Geometry: final body of the model. Coordinates: model frame, mm. Give positions to 0.01 mm unless a question says otherwise; leave off trailing zeros. Write each loop counter-clockwise with the first axis right and the second up, starting at its lowest first coordinate (ties: lowest second). Pieces come first, ordered by that corner, then holes.
from build123d import *

# Parameters (mm, degrees)
SKETCH_1_W      = 228
SKETCH_1_H      = 84
SKETCH_1_R      = 5
SKETCH_1_R_2    = 1.65
SKETCH_1_R_3    = 2.15
EXTRUDE_1_DEPTH = 1


with BuildPart() as part:
    # Эскиз1 → Вытянуть1 (new body)
    with BuildSketch(Plane.XY):
        Rectangle(SKETCH_1_W, SKETCH_1_H)
        with Locations((74, -2)):
            Circle(SKETCH_1_R, mode=Mode.SUBTRACT)
        with Locations((74, -12)):
            Circle(SKETCH_1_R_2, mode=Mode.SUBTRACT)
        with Locations((62, -2)):
            Circle(SKETCH_1_R, mode=Mode.SUBTRACT)
        with Locations((62, -12)):
            Circle(SKETCH_1_R_2, mode=Mode.SUBTRACT)
        with Locations((50, -2)):
            Circle(SKETCH_1_R, mode=Mode.SUBTRACT)
        with Locations((50, -12)):
            Circle(SKETCH_1_R_2, mode=Mode.SUBTRACT)
        with Locations((38, -2)):
            Circle(SKETCH_1_R, mode=Mode.SUBTRACT)
        with Locations((38, -12)):
            Circle(SKETCH_1_R_2, mode=Mode.SUBTRACT)
        with Locations((107, 32)):
            Circle(SKETCH_1_R_3, mode=Mode.SUBTRACT)
        with Locations(Location((-107, 32, 0), (0, 0, 180))):
            Circle(SKETCH_1_R_3, mode=Mode.SUBTRACT)
        with Locations((-107, -32)):
            Circle(SKETCH_1_R_3, mode=Mode.SUBTRACT)
        with Locations(Location((107, -32, 0), (0, 0, 180))):
            Circle(SKETCH_1_R_3, mode=Mode.SUBTRACT)
    extrude(amount=EXTRUDE_1_DEPTH)


solid = part.part
Q1. Pull-direction query (Y, two-part tool) for faces 1 (the cylindrical face through (108.585, -33.453, 0.493)), 2 (the flat face through (-2, 1, 0)); classes: released by +Y, released by -Y, zero draft, split by the parting line, or undercut.
Filled sheet:
face 1: undercut
face 2: zero draft
Q2. Section A-A on x = -107. Output: boundary loops of the cut face in (y, z), plus the area to 3 significant figures.
Filled sheet:
outline: (-42, 0) - (-34.15, 0) - (-34.15, 1) - (-42, 1) - close; (-29.85, 0) - (29.85, 0) - (29.85, 1) - (-29.85, 1) - close; (34.15, 0) - (42, 0) - (42, 1) - (34.15, 1) - close
area: 75.4 mm2
Q3. Pin query (flat end, axial travel): P1, Ø16, axis at x = 38, y = -2, coming from the +Z side; P2, Ø4, axis at x = -107, y = 32, coming from the +Z side. Return the tip coordinate at first contact, or that it passes through.
Filled sheet:
P1: stops at z = 1
P2: passes through
Q4. Ray query, line 1 along Y through (x, z) = (50, 0.75); line 2 along Y through (x, z) = (107, 0.45); line 3 along X through (y, z) = (-10.5, 0.9). Return the intervals inside material, ascending.
Filled sheet:
line 1: y = -42 to -13.65, -10.35 to -7, 3 to 42
line 2: y = -42 to -34.15, -29.85 to 29.85, 34.15 to 42
line 3: x = -114 to 37.31, 38.69 to 49.31, 50.69 to 61.31, 62.69 to 73.31, 74.69 to 114
Q5. Section B-B on z = 0.4. Count the separate pieces of the cut face and the enclosed holes in it, plus the area to 3 significant figures.
Filled sheet:
separate pieces: 1
enclosed holes: 12
area: 18,700 mm2
